```python
from build123d import *

# Parameters (mm, degrees)
F0_W     = 38.1
F0_H     = 44.45
F1_DEPTH = 25.4
F2_W     = 12.7
F2_H     = 10.368286
F3_DEPTH = 25.401
F5_DEPTH = 25.401


with BuildPart() as f1:
    # F0 (on Front) → F1 (new body)
    with BuildSketch(Plane.XZ):
        with Locations((-48.974418, 32.146238)):
            Rectangle(F0_W, F0_H)
    extrude(amount=F1_DEPTH)

    # F2 (on face) → F3 (cut, through all)
    with BuildSketch(Plane.XZ.offset(25.4)):
        with Locations((-48.974418, 15.105381)):
            Rectangle(F2_W, F2_H)
    extrude(amount=-F3_DEPTH, mode=Mode.SUBTRACT)

    # F4 (on face) → F5 (cut, through all)
    with BuildSketch(Plane.XZ.offset(25.4)):
        Polygon((-68.024418, 54.371238), (-68.024418, 9.921238), (-55.324418, 54.371238), align=None)
        Polygon((-29.924418, 54.371238), (-42.624418, 54.371238), (-29.924418, 9.921238), align=None)
    extrude(amount=-F5_DEPTH, mode=Mode.SUBTRACT)


solid = f1.part
```
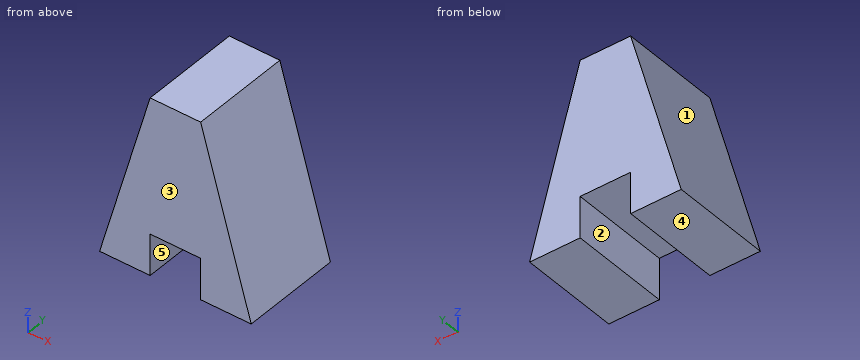
Design review of the part built by this model. Coordinates are the model's own, in mm. Face numbers are marked on the shaded views. A direction names the side the tool comes from. Round coordinates to 2 decimals unless told otherwise and drop trailing zeros. Write each loop counter-clockwise with the first axis right and the second up, starting at its lowest first coordinate (ties: lowest second). Pieces come first, ordered by that corner, then holes. Notation, with made-up numbers: (0, 25) -> (15, 25) arc R14 ccw to (15, 44) -> close; hole circle Ø11 at (-30.75, 37.5). An arc over 180 degrees is marked (long way). Write item = value, one per line. Start each with the question number.
1) Tool access review of the marked faces 4 and 5: name each direction out of +Z, -Z, +X, -X, +Y, -Y from which nothing blocks a thin tool from reaching the whole face with its end or side.
2) Take a section at C-C, the plane x = -48. State the section outline as (y, z) points.
3) Clearance check with flat-ended pins moving along their axes: pin 1 (12 mm diameter, centred on y = -10.5, z = 31.5, fed in from -X); pin 2 (5 mm diameter, centred on y = -14.5, z = 15, fed in from +X); pin 3 (8.5 mm diameter, centred on y = -18.5, z = 16, fed in from -X). State where each tip first meets the part, or that it passes through.
4) Take a section at A-A, the plane y = -7.25. State the section outline as (x, z) points.
5) Mouldability with a two-part tool opening along X and no side actions: class the marked faces 1, 2 and 3 as +X half, -X half, draft (parallel to the pull), parting line (faces both ways), or undercut.
6) Take a section at B-B, the plane z = 19. State the section outline as (x, y) points.
7) Wall thickness on probe 1 along Z at (x, y) = (-47, -21.25); probe 2 along X at (y, z) = (-16.75, 19.5); probe 3 along X at (y, z) = (-6.5, 18): over which ranges is each line inside the solid? List them lowest first. Write a range as from..to.
8) Take a section at D-D, the plane z = 39.5. State the section outline as (x, y) points, plus the area to 3 significant figures.
Results list:
q1.face_4 = -Z, +X, -X, +Y, -Y
q1.face_5 = -Z, +Y, -Y
q2.outline = (-25.4, 20.29) -> (0, 20.29) -> (0, 54.37) -> (-25.4, 54.37) -> close
q3.pin_1 = -63.57
q3.pin_2 = -30.66
q3.pin_3 = -67.5
q4.outline = (-68.02, 9.92) -> (-55.32, 9.92) -> (-55.32, 20.29) -> (-42.62, 20.29) -> (-42.62, 9.92) -> (-29.92, 9.92) -> (-42.62, 54.37) -> (-55.32, 54.37) -> close
q5.face_1 = -X half
q5.face_2 = undercut
q5.face_3 = draft
q6.outline = (-65.43, -25.4) -> (-55.32, -25.4) -> (-55.32, 0) -> (-65.43, 0) -> close; (-42.62, -25.4) -> (-32.52, -25.4) -> (-32.52, 0) -> (-42.62, 0) -> close
q7.probe_1 = 20.29..54.37
q7.probe_2 = -65.29..-55.32, -42.62..-32.66
q7.probe_3 = -65.72..-55.32, -42.62..-32.23
q8.outline = (-59.57, -25.4) -> (-38.38, -25.4) -> (-38.38, 0) -> (-59.57, 0) -> close
q8.area = 538 mm²
